The listing builds one solid part. Answer for the finished solid, in the listing's coordinates (mm). Face numbers are marked on the shaded views. A direction names the side the tool comes from. Coordinates: 2 decimals unless noted, no trailing zeros. Order: outer loops, then holes, each group sorted by start corner. A loop starts at its lowest first (then second) coordinate and runs counter-clockwise, first axis right, second up. Notation, with made-up numbers: (-15.5, 78) -> (8.5, 78) arc R15 cw to (8.5, 101) -> close; hole circle Ø3 at (62, -40). An arc over 180 degrees is marked (long way). Return JSON: item names as keys, results as strings.
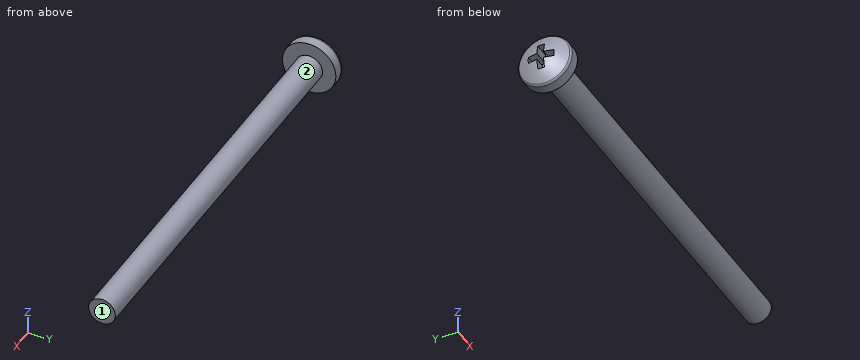
```python
from build123d import *

# Parameters (mm, degrees)
CUT_EXTRUDE4_DEPTH = 2.5


with BuildPart() as part:
    # Sketch1 → Revolve1 (revolve)
    with BuildSketch(Plane.XY, mode=Mode.PRIVATE) as revolve1_sk:
        with BuildLine():
            Line((3.1, 2), (3.1, 4))
            Line((3.1, 4), (1.616353821, 4))
            ThreePointArc((1.616353821, 4), (1.397629036, 3.947269784), (1.226960106, 3.800664452))
            ThreePointArc((1.226960106, 3.800664452), (0.314340807, 1.996902688), (0, 0))
            Line((0, 0), (63.1, 0))
            Line((63.1, 0), (63.1, 2))
            Line((63.1, 2), (3.1, 2))
        make_face()
    revolve(revolve1_sk.sketch.rotate(Axis((63.1, 0, 0), (-1, 0, 0)), 90), axis=Axis((63.1, 0, 0), (-1, 0, 0)))

    # Sketch2 → Cut-Extrude4 (cut)
    with BuildSketch(Plane(origin=(0, 0, 0), x_dir=(0, 0, -1), z_dir=(1, 0, 0))):
        Polygon((-0.5, -0.5), (-0.5, -1.936491673), (0.5, -1.936491673), (0.5, -0.5), (1.936491673, -0.5), (1.936491673, 0.5), (0.5, 0.5), (0.5, 1.936491673), (-0.5, 1.936491673), (-0.5, 0.5), (-1.936491673, 0.5), (-1.936491673, -0.5), align=None)
    extrude(amount=CUT_EXTRUDE4_DEPTH, mode=Mode.SUBTRACT)


solid = part.part
```
Item 1: Flat-ended cylindrical pins translate along their axes: pin 1 (0.8 mm diameter, centred on x = 1, y = 0, fed in from -Z); pin 2 (2 mm diameter, centred on x = 10.5, z = 2, fed in from -Y); pin 3 (0.7 mm diameter, centred on x = 1, y = 1.5, fed in from -Z). Find the tip coordinate at first contact, or state that the pin passes through.
Answer list:
{"pin 1": "z = -3.95", "pin 2": "y = -1.73", "pin 3": "z = -3.65"}
Item 2: Which of the six approach directions +Z, -Z, +X, -X, +Y, -Y give full straight-line access (tool end or side, diameter ignored) to the marked faces 1 and 2?
Answer list:
{"face 1": "+Z, -Z, +X, +Y, -Y", "face 2": "+X"}
Item 3: The part is cut by section A-A on x = 39. Determine the outline of the cut face in (y, z).
Answer list:
{"outline": "circle Ø4 at (0, 0)"}
Item 4: Find the intervals of material crossed by probe 1 along Y at (x, z) = (33, 0); probe 2 along X at (y, z) = (0.75, 3.25); probe 3 along X at (y, z) = (0.5, 2), in increasing order.
Answer list:
{"probe 1": "-2 to 2", "probe 2": "0.92 to 3.1", "probe 3": "0.34 to 3.1"}
